Verification items for the finished model (mm, model axes). Face numbers are marked on the shaded views. A direction names the side the tool comes from. Coordinates: 2 decimals unless noted, no trailing zeros. Write each loop counter-clockwise with the first axis right and the second up, starting at its lowest first coordinate (ties: lowest second). Pieces come first, ordered by that corner, then holes. Notation, with made-up numbers: (2, -14.75) - (50, -14.75) arc R27 cw to (50, 15.25) - close; hole circle Ø9 at (31, 37). An arc over 180 degrees is marked (long way). Use CSV: the item, a comma, the result in double quotes. Start each with the question number.
```python
from build123d import *

# Parameters (mm, degrees)
SKETCH1_R           = 10.16
BOSS_EXTRUDE2_DEPTH = 3.175
SKETCH4_R           = 6.35
BOSS_EXTRUDE3_DEPTH = 6.35
SKETCH5_R           = 4.7625
CUT_EXTRUDE3_DEPTH  = 6.35
SKETCH6_R           = 1.1303
CUT_EXTRUDE4_DEPTH  = 16.709032434


with BuildPart() as part:
    # Sketch1 → Boss-Extrude2 (new body)
    with BuildSketch(Plane.XY):
        Circle(SKETCH1_R)
    extrude(amount=BOSS_EXTRUDE2_DEPTH)

    # Sketch4 → Boss-Extrude3 (add)
    with BuildSketch(Plane.XY.offset(3.175)):
        Circle(SKETCH4_R)
    extrude(amount=BOSS_EXTRUDE3_DEPTH)

    # Sketch5 → Cut-Extrude3 (cut)
    with BuildSketch(Plane(origin=(0, 0, 0), x_dir=(-1, 0, 0), z_dir=(0, 0, -1))):
        Circle(SKETCH5_R)
    extrude(amount=-CUT_EXTRUDE3_DEPTH, mode=Mode.SUBTRACT)

    # Sketch6 → Cut-Extrude4 (cut, through all)
    with BuildSketch(Plane.XY.offset(3.175)):
        with Locations((0, 8.255)):
            Circle(SKETCH6_R)
        with Locations((0, -8.255)):
            Circle(SKETCH6_R)
    extrude(amount=-CUT_EXTRUDE4_DEPTH, mode=Mode.SUBTRACT)


solid = part.part
```
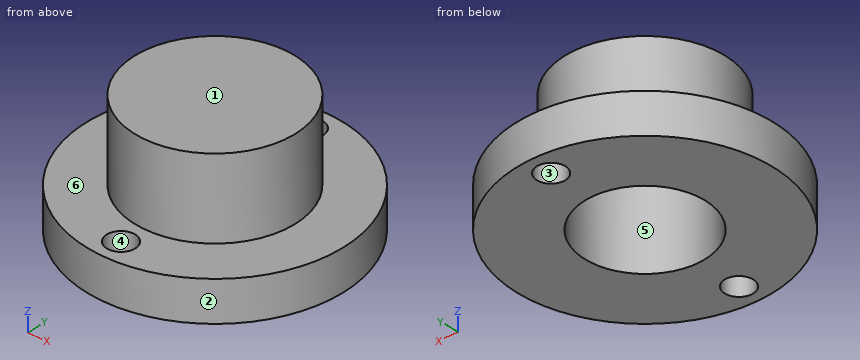
Q1. Cross-section at D-D (x = -3). Record the cut outline in (y, z) (3 decimals).
Q2. Gauge pin test, flat ends, axial feed: pin 1 (1.5 mm diameter, centred on x = 3, z = 2, fed in from +Y); pin 2 (1.4 mm diameter, centred on x = 0, y = -8.255, fed in from +Z); pin 3 (4 mm diameter, centred on x = 6.5, z = 2, fed in from +Y); pin 4 (7.5 mm diameter, centred on x = -0.5, y = 0.5, fed in from -Z). Record the tip position at first contact, or that the pin passes through.
Q3. Cross-section at B-B (y = -7.75). Record the cut outline in (x, z) (3 decimals).
Q4. Cross-section at A-A (x = 0). State how many separate pieces and enclosed holes the cut face has, plus the area to 3 significant figures.
Q5. Release check for a two-part mould opening along X. For the marked faces 1, 2 and 3 record: released by +X, released by -X, zero draft, split by the parting line, or undercut.
Q6. Tool access check on the marked faces 4, 5 and 6. Record the directions out of +Z, -Z, +X, -X, +Y, -Y that give a thin tool (end or side, any length) a straight path to the whole face; none if there is none.
Q7. Scan lines: line 1 along Y through (x, z) = (0, 1.8); line 2 along Z through (x, y) = (-8, -0.5) (3 decimals); line 3 along Y through (x, z) = (-1, 1). Record each from-to range of solid material in increasing order. Write a range as from..to.
Reply:
1,outline,"(-9.707, 0) - (-3.699, 0) - (-3.699, 6.35) - (3.699, 6.35) - (3.699, 0) - (9.707, 0) - (9.707, 3.175) - (5.597, 3.175) - (5.597, 9.525) - (-5.597, 9.525) - (-5.597, 3.175) - (-9.707, 3.175) - close"
2,pin 1,"y = 9.91"
2,pin 2,"through"
2,pin 3,"y = 9.11"
2,pin 4,"z = 6.35"
3,outline,"(-6.57, 0) - (-1.011, 0) - (-1.011, 3.175) - (-6.57, 3.175) - close; (1.011, 0) - (6.57, 0) - (6.57, 3.175) - (1.011, 3.175) - close"
4,separate pieces,"3"
4,enclosed holes,"0"
4,area,"70.3 mm^2"
5,face 1,"zero draft"
5,face 2,"split by the parting line"
5,face 3,"undercut"
6,face 4,"+Z, -Z"
6,face 5,"-Z"
6,face 6,"+Z"
7,line 1,"-10.16..-9.39, -7.12..-4.76, 4.76..7.12, 9.39..10.16"
7,line 2,"0..3.175"
7,line 3,"-10.11..-8.78, -7.73..-4.66, 4.66..7.73, 8.78..10.11"
